Check sheet for the modelled part. Datum: model origin and axes. Units: mm. Face numbers are marked on the shaded views. A direction names the side the tool comes from. Round coordinates to 2 decimals unless told otherwise and drop trailing zeros. Write each loop counter-clockwise with the first axis right and the second up, starting at its lowest first coordinate (ties: lowest second). Pieces come first, ordered by that corner, then holes. Notation, with made-up numbers: (35, -31) - (92, -31) arc R23 cw to (92, -13) - close; hole circle Ø5 at (16, 13.25). An arc over 180 degrees is marked (long way). Answer as a JSON object with one key per item and string values. Group by question number.
Item 1: Gauge pin test, flat ends, axial feed: P1, Ø1.4, axis at x = 0, y = -7.5, coming from the -Z side; P2, Ø2.5, axis at y = -4, z = 16.5, coming from the +X side; P3, Ø3, axis at x = 0.5, y = -7.5, coming from the +Z side; P4, Ø1.5, axis at y = -3.5, z = 28.5, coming from the -X side. Record the tip position at first contact, or that the pin passes through.
Item 2: Thickness scan on line 1 (Z direction, x = 0, y = -0.7); line 2 (Z direction, x = 0.75, y = -1); line 3 (Y direction, x = 1.25, z = 3). Record the ranges inside material, lowest first.
Item 3: Sectioned sample at B-B on y = -6. Record the boundary of the cut face in (x, z), plus the area to 3 significant figures.
Item 4: Sectioned sample at C-C on z = 23. Record the boundary of the cut face in (x, y).
Item 5: Sectioned sample at D-D on x = 4. Record the boundary of the cut face in (y, z).
Item 6: Sectioned sample at A-A on x = 0. Record the boundary of the cut face in (y, z).
Item 7: Release check for a two-part mould opening along X. For the marked faces 4, 5 and 6 record: pulls with the +X half, pulls with the -X half, needs draft (parallel to the pull), parting line crosses it, or undercut.
Item 8: Set-up check for the marked faces 1, 2 and 3: record each of +Z, -Z, +X, -X, +Y, -Y from which the full face is reachable in a straight line by a thin tool's end or side.
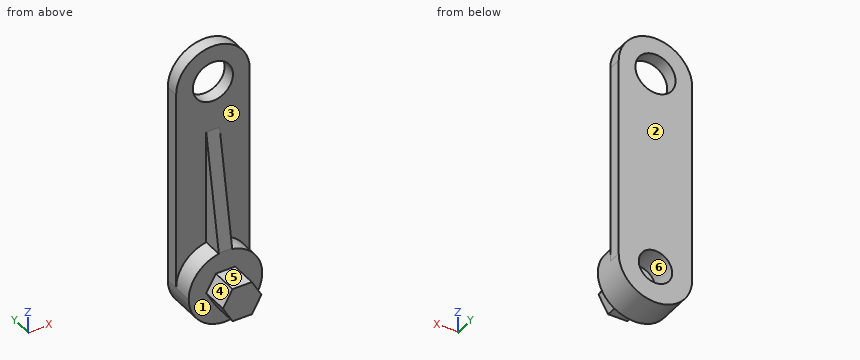
```python
from build123d import *

# Parameters (mm, degrees)
F0_R     = 3
F1_DEPTH = 2
F2_DEPTH = 5
F3_DEPTH = 9
F5_DEPTH = 1
F6_W     = 4
F6_H     = 2.5


with BuildPart() as f1:
    # F0 (on Front) → F1 (new body)
    with BuildSketch(Plane.XZ):
        with BuildLine():
            ThreePointArc((5.5, 30), (0, 35.5), (-5.5, 30))
            Line((-5.5, 30), (-5.5, 0))
            ThreePointArc((-5.5, 0), (0, 5.5), (5.5, 0))
            Line((5.5, 0), (5.5, 30))
        make_face()
        with Locations((0, 30)):
            Circle(F0_R, mode=Mode.SUBTRACT)
    extrude(amount=F1_DEPTH)

    # F0 (on Front) → F2 (join)
    with BuildSketch(Plane.XZ):
        with BuildLine():
            ThreePointArc((5.5, 0), (0, 5.5), (-5.5, 0))
            ThreePointArc((-5.5, 0), (0, -5.5), (5.5, 0))
        make_face()
        Polygon((-2.886751, 0), (-1.443376, 2.5), (1.443376, 2.5), (2.886751, 0), (1.443376, -2.5), (-1.443376, -2.5), align=None, mode=Mode.SUBTRACT)
    extrude(amount=F2_DEPTH)

    # F0 (on Front) → F3 (join)
    with BuildSketch(Plane.XZ):
        Polygon((1.443376, 2.5), (-1.443376, 2.5), (-2.886751, 0), (-1.443376, -2.5), (1.443376, -2.5), (2.886751, 0), align=None)
    extrude(amount=F3_DEPTH)

    # F4 (on Right) → F5 (join, symmetric)
    with BuildSketch(Plane.YZ):
        Polygon((-5, 5.5), (-5, 3.5), (-2, 3.5), (-2, 5.5), (-2, 22.513845), align=None)
    extrude(amount=F5_DEPTH, both=True)

    # F6 (on Right) → F7 (revolve, cut)
    with BuildSketch(Plane.YZ):
        with Locations((-2, 1.25)):
            Rectangle(F6_W, F6_H)
    revolve(axis=Axis((0, -2, 0), (0, -1, 0)), mode=Mode.SUBTRACT)


solid = f1.part
```
Completed:
{
 "1": {"P1": "z = -2.5", "P2": "x = 1", "P3": "z = 2.5", "P4": "through"},
 "2": {"line 1": "-5.5 to -2.5, 2.5 to 27, 33 to 35.5", "line 2": "-5.45 to -2.38, 2.38 to 27.1, 32.9 to 35.45", "line 3": "-5 to 0"},
 "3": {"outline": "(-2.89, 0) - (-1.44, -2.5) - (1.44, -2.5) - (2.89, 0) - (1.44, 2.5) - (-1.44, 2.5) - close", "area": "21.7 mm²"},
 "4": {"outline": "(-5.5, -2) - (5.5, -2) - (5.5, 0) - (-5.5, 0) - close"},
 "5": {"outline": "(-5, -3.77) - (0, -3.77) - (0, 33.77) - (-2, 33.77) - (-2, 3.77) - (-5, 3.77) - close"},
 "6": {"outline": "(-9, -2.5) - (-5, -2.5) - (-5, -5.5) - (0, -5.5) - (0, -2.5) - (-4, -2.5) - (-4, 2.5) - (0, 2.5) - (0, 27) - (-2, 27) - (-2, 22.51) - (-5, 5.5) - (-5, 2.5) - (-9, 2.5) - close; (-2, 33) - (0, 33) - (0, 35.5) - (-2, 35.5) - close"},
 "7": {"face 4": "pulls with the -X half", "face 5": "needs draft", "face 6": "undercut"},
 "8": {"face 1": "-Y", "face 2": "+Z, -Z, +X, -X, +Y", "face 3": "+Z, -Y"}
}
